For this review, take the finished solid that the model builds, in its own axes (mm). A direction names the side the tool comes from. Give positions to 0.01 mm unless a question says otherwise; leave off trailing zeros. Write each loop counter-clockwise with the first axis right and the second up, starting at its lowest first coordinate (ties: lowest second). Pieces come first, ordered by that corner, then holes. Notation, with made-up numbers: (8, -23.5) -> (44, -23.5) arc R18 cw to (44, 10.5) -> close; hole circle Ø11 at (-28.5, 15). An arc over 180 degrees is marked (long way). Write item = value, one per line.
```python
from build123d import *
from build123d.topology import SkipClean

# Parameters (mm, degrees)
SKETCH3_R           = 43
BOSS_EXTRUDE2_DEPTH = 15.5
BOSS_EXTRUDE5_DEPTH = 10
SKETCH9_W           = 75.940248911
SKETCH9_H           = 24.034829181
CUT_EXTRUDE8_DEPTH  = 20
SKETCH10_R          = 5
CUT_EXTRUDE9_DEPTH  = 20
SKETCH11_R          = 5
CUT_EXTRUDE10_DEPTH = 20


with BuildPart() as part:
    # Sketch3 → Boss-Extrude2 (new body)
    with BuildSketch(Plane(origin=(0, 0, 0), x_dir=(1, 0, 0), z_dir=(0, 1, 0))):
        with Locations(Location((0, 0, 0), (0, 0, 270))):
            Circle(SKETCH3_R)
    extrude(amount=BOSS_EXTRUDE2_DEPTH)

    # Sketch4 → Boss-Extrude5 (add)
    with SkipClean():  # the faces are left unmerged after this step: merging them gives an invalid solid
        with BuildSketch(Plane(origin=(0, 15.5, 0), x_dir=(1, 0, 0), z_dir=(0, 1, 0))):
            with BuildLine():
                Line((-38.065732621, 20), (-32.310988843, 20))
                ThreePointArc((-32.310988843, 20), (-38, 0), (-32.310988843, -20))
                Line((-32.310988843, -20), (-38.065732621, -20))
                ThreePointArc((-38.065732621, -20), (-43, 0), (-38.065732621, 20))
            make_face()
            with BuildLine():
                Line((32.310988843, 20), (38.065732621, 20))
                ThreePointArc((38.065732621, 20), (43, 0), (38.065732621, -20))
                Line((38.065732621, -20), (32.310988843, -20))
                ThreePointArc((32.310988843, -20), (38, 0), (32.310988843, 20))
            make_face()
        extrude(amount=BOSS_EXTRUDE5_DEPTH)

    # Sketch9 → Cut-Extrude8 (cut)
    with BuildSketch(Plane(origin=(0, 15.5, 0), x_dir=(1, 0, 0), z_dir=(0, 1, 0))):
        with Locations((-0.095608165, -32.01741459)):
            Rectangle(SKETCH9_W, SKETCH9_H)
        with Locations((-0.095608165, 32.01741459)):
            Rectangle(SKETCH9_W, SKETCH9_H)
    extrude(amount=-CUT_EXTRUDE8_DEPTH, mode=Mode.SUBTRACT)

    # Sketch10 → Cut-Extrude9 (cut)
    with BuildSketch(Plane.XZ):
        with Locations(Location((0, 0, 0), (0, 0, 270))):
            Circle(SKETCH10_R)
    extrude(amount=-CUT_EXTRUDE9_DEPTH, mode=Mode.SUBTRACT)

    # Sketch11 → Cut-Extrude10 (cut)
    with BuildSketch(Plane.XZ):
        with Locations(Location((25, 0, 0), (0, 0, 270))):
            Circle(SKETCH11_R)
        with Locations(Location((-25, 0, 0), (0, 0, 90))):
            Circle(SKETCH11_R)
    extrude(amount=-CUT_EXTRUDE10_DEPTH, mode=Mode.SUBTRACT)


solid = part.part
```
(1) Tool access review of faces 1 (the face through (-38, 20, 0)), 2 (the face through (20.12, 7.64, 1.08)): name each direction out of +Z, -Z, +X, -X, +Y, -Y from which nothing blocks a thin tool from reaching the whole face with its end or side.
Answers below:
face_1 = +Y
face_2 = +Y, -Y
(2) Take a section at A-A (x = -25). Write out the cut boundary in (y, z), plus the area to 3 significant figures.
Answers below:
outline = (0, -20) -> (15.5, -20) -> (15.5, -5) -> (0, -5) -> close; (0, 5) -> (15.5, 5) -> (15.5, 20) -> (0, 20) -> close
area = 465 mm^2
(3) Take a section at D-D (y = 12). Write out the cut boundary in (x, z).
Answers below:
outline = (-38.07, -20) -> (37.87, -20) -> (37.87, -20.36) arc R43 ccw to (37.87, 20.36) -> (37.87, 20) -> (-38.07, 20) arc R43 ccw to start; hole circle Ø10 at (-25, 0); hole circle Ø10 at (0, 0); hole circle Ø10 at (25, 0)
(4) To check wall thickness, follow probe 1 along X at (y, z) = (9.25, 0); probe 2 along Y at (x, z) = (16.5, 17.5); probe 3 along Z at (x, y) = (29, 3). State the ranges of each line that lie inside material, in increasing order.
Answers below:
probe_1 = -43 to -30, -20 to -5, 5 to 20, 30 to 43
probe_2 = 0 to 15.5
probe_3 = -20 to -3, 3 to 20
(5) Take a section at B-B (y = 17.5). Write out the cut boundary in (x, z).
Answers below:
outline = (-38.07, -20) -> (-32.31, -20) arc R38 cw to (-32.31, 20) -> (-38.07, 20) arc R43 ccw to start; (32.31, -20) -> (38.07, -20) arc R43 ccw to (38.07, 20) -> (32.31, 20) arc R38 cw to start
(6) For pin 1 (8 mm diameter, centred on x = 30.5, y = 3.5, fed in from -Z); pin 2 (13 mm diameter, centred on x = 4.5, y = 17, fed in from +Z); pin 3 (2 mm diameter, centred on x = -11, z = -13.5, fed in from +Y); pin 4 (6 mm diameter, centred on x = -25, z = 0, fed in from -Y), all flat-tipped, find the tip position at first contact; note any pin that passes through.
Answers below:
pin_1 = -20
pin_2 = 20
pin_3 = 15.5
pin_4 = through
(7) The part is to be moulded in two halves that separate along Z. For faces 3 (the face through (-39, 25.5, 0)), 4 (the face through (-1, 10, -20)), 5 (the face through (38, 20, 0)), say which applies: released by +Z, released by -Z, zero draft, split by the parting line, or undercut.
Answers below:
face_3 = zero draft
face_4 = released by -Z
face_5 = undercut
(8) Take a section at C-C (z = 0). Write out the cut boundary in (x, y), plus the area to 3 significant figures.
Answers below:
outline = (-43, 0) -> (-30, 0) -> (-30, 15.5) -> (-38, 15.5) -> (-38, 25.5) -> (-43, 25.5) -> close; (-20, 0) -> (-5, 0) -> (-5, 15.5) -> (-20, 15.5) -> close; (5, 0) -> (20, 0) -> (20, 15.5) -> (5, 15.5) -> close; (30, 0) -> (43, 0) -> (43, 25.5) -> (38, 25.5) -> (38, 15.5) -> (30, 15.5) -> close
area = 968 mm^2
